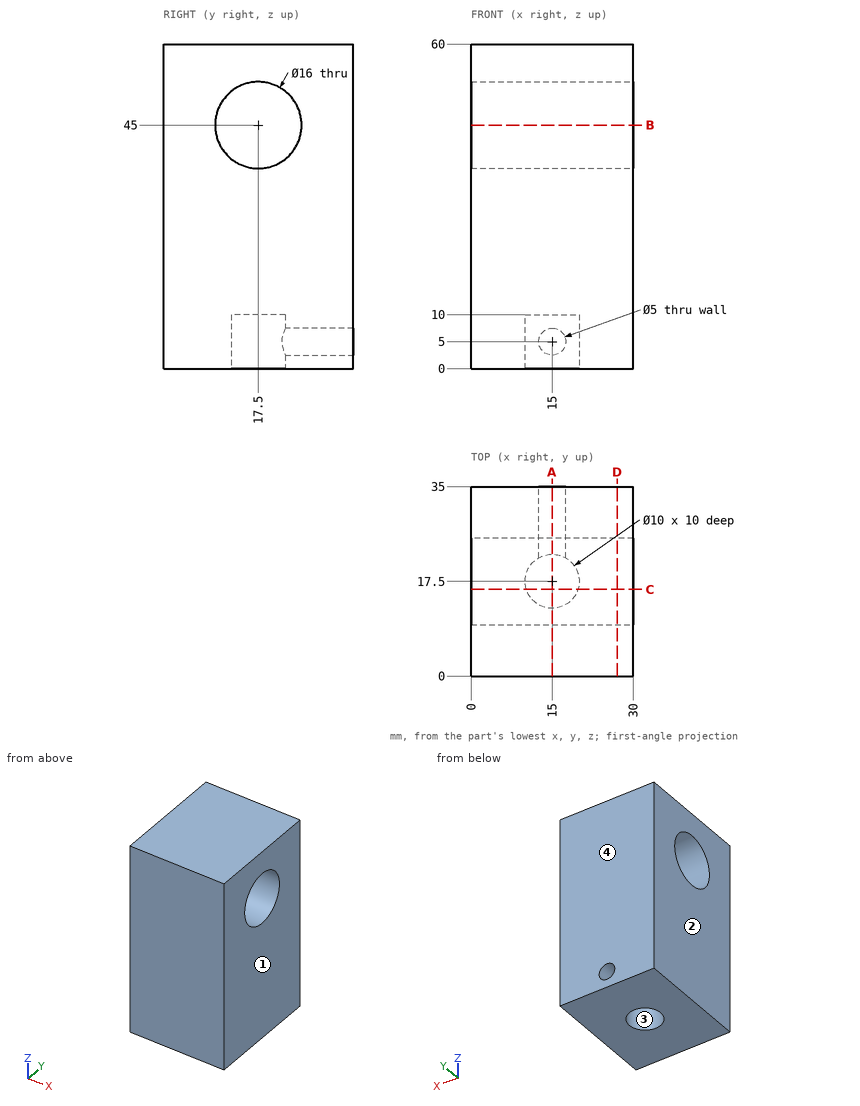
Source: three-view drawing plus pictorial views. Frame: mm from the lowest corner of the part. Round coordinates to 2 decimals unless told otherwise and drop trailing zeros. Write each loop counter-clockwise with the first axis right and the second up, starting at its lowest first coordinate (ties: lowest second). Pieces come first, ordered by that corner, then holes. Notation, with made-up numbers: (-8.75, 4.25) -> (12.25, 4.25) arc R32 cw to (12.25, 33.25) -> close; hole circle Ø8 at (58, 70). An arc over 180 degrees is marked (long way). Return JSON: item names as keys, results as strings.
Q1. Section D-D on x = 27. Return the cut outline in (y, z).
From the geometry:
{"outline": "(0, 0) -> (35, 0) -> (35, 60) -> (0, 60) -> close; hole circle Ø16 at (17.5, 45)"}
Q2. First-contact query: pin 1 Ø6 at (y, z) = (22, 45) entering from +X; pin 2 Ø5 at (x, y) = (15, 16) entering from -Z. Flat tips, straight axial feed; report the tip coordinate or a pass-through.
From the geometry:
{"pin 1": "through", "pin 2": "z = 10"}
Q3. Ray query, line 1 (Z direction, x = 15, y = 30.25); line 2 (Z direction, x = 15, y = 24.5); line 3 (Z direction, x = 13, y = 17.5). Return the intervals inside material, ascending.
From the geometry:
{"line 1": "0 to 2.5, 7.5 to 60", "line 2": "0 to 2.5, 7.5 to 41.13, 48.87 to 60", "line 3": "10 to 37, 53 to 60"}
Q4. Section B-B on z = 45. Return the cut outline in (x, y).
From the geometry:
{"outline": "(0, 0) -> (30, 0) -> (30, 9.5) -> (0, 9.5) -> close; (0, 25.5) -> (30, 25.5) -> (30, 35) -> (0, 35) -> close"}
Q5. Section A-A on x = 15. Return the cut outline in (y, z), and give its area (3 significant figures).
From the geometry:
{"outline": "(0, 0) -> (12.5, 0) -> (12.5, 10) -> (22.5, 10) -> (22.5, 7.5) -> (35, 7.5) -> (35, 60) -> (0, 60) -> close; (22.5, 0) -> (35, 0) -> (35, 2.5) -> (22.5, 2.5) -> close; hole circle Ø16 at (17.5, 45)", "area": "1,740 mm2"}
Q6. Section C-C on y = 16. Return the cut outline in (x, z), and give its area (3 significant figures).
From the geometry:
{"outline": "(0, 0) -> (10.23, 0) -> (10.23, 10) -> (19.77, 10) -> (19.77, 0) -> (30, 0) -> (30, 37.14) -> (0, 37.14) -> close; (0, 52.86) -> (30, 52.86) -> (30, 60) -> (0, 60) -> close", "area": "1,230 mm2"}
Q7. Mould query, pull axis X, two halves, no side actions, for the marked faces 1, 2, 3 and 4. Classes: +X half, -X half, draft (parallel to the pull), parting line (faces both ways), or undercut.
From the geometry:
{"face 1": "+X half", "face 2": "-X half", "face 3": "undercut", "face 4": "draft"}
